```python
from build123d import *

# Parameters (mm, degrees)
F0_W          = 279.4
F0_H          = 6.35
F1_DEPTH      = 127
F1_DEPTH_BACK = 127
F2_W          = 76.2
F2_H          = 6.35
F3_DEPTH      = 82.55
F4_W          = 57.15
F4_H          = 6.35
F5_DEPTH      = 69.85
F6_R          = 1.5875
F7_DEPTH      = 6.351
F8_R          = 1.5875
F9_DEPTH      = 6.351


with BuildPart() as f1:
    # F0 (on Top) → F1 (new body, two sides)
    with BuildSketch(Plane.XY) as f1_sk:
        Rectangle(F0_W, F0_H)
    extrude(amount=F1_DEPTH)
    extrude(f1_sk.sketch, amount=-F1_DEPTH_BACK)

    # F0 (on Top) + F2 (on face) → F3 (join)
    with BuildSketch(Plane.XY):
        Rectangle(F0_W, F0_H)
    with BuildSketch(Plane.XY.offset(127)):
        Rectangle(F2_W, F2_H)
    extrude(amount=F3_DEPTH)

    # F4 (on face) → F5 (join)
    with BuildSketch(Plane(origin=(0, 0, -127), x_dir=(1, 0, 0), z_dir=(0, 0, -1))):
        Rectangle(F4_W, F4_H)
    extrude(amount=F5_DEPTH)

    # F6 (on face) → F7 (cut, through all)
    with BuildSketch(Plane.XZ.offset(3.175)):
        with Locations((-17.4625, -171.45)):
            Circle(F6_R)
        with Locations((17.4625, -171.45)):
            Circle(F6_R)
    extrude(amount=-F7_DEPTH, mode=Mode.SUBTRACT)

    # F8 (on face) → F9 (cut, through all)
    with BuildSketch(Plane.XZ.offset(3.175)):
        with Locations((-15.08125, 177.8)):
            Circle(F8_R)
        with Locations((15.08125, 177.8)):
            Circle(F8_R)
    extrude(amount=-F9_DEPTH, mode=Mode.SUBTRACT)


solid = f1.part
```
Work out the finished part from the listing and answer in its coordinate system (mm). Coordinates: 2 decimals unless noted, no trailing zeros. Order: outer loops, then holes, each group sorted by start corner. A loop starts at its lowest first (then second) coordinate and runs counter-clockwise, first axis right, second up. Notation, with made-up numbers: (28, 38) - (72, 38) arc R23 ccw to (72, 55) - close; hole circle Ø7 at (-6.5, 69.25). An arc over 180 degrees is marked (long way). Answer as a JSON object with one key per item and string values.
1. Find section B-B on x = 117.5. Determine the outline of the cut face in (y, z) (3 decimals).
Output values:
{"outline": "(-3.175, -127) - (3.175, -127) - (3.175, 127) - (-3.175, 127) - close"}
2. Find section A-A on y = -1. Count the separate pieces of the cut face and the enclosed holes in it, plus the area to 3 significant figures.
Output values:
{"separate pieces": "1", "enclosed holes": "4", "area": "81,200 mm²"}
3. Each of these flat-tipped pins is pushed along its axis until it touches: P1, Ø3, axis at x = -104, y = -1, coming from the -Z side; P2, Ø1, axis at y = 2, z = 164.5, coming from the -X side; P3, Ø1.9, axis at x = 112.5, y = 0.5, coming from the +Z side; P4, Ø3, axis at x = 15.08, z = 177.8, coming from the +Y side. Where does it stop, or does it pass through?
Output values:
{"P1": "stops at z = -127", "P2": "stops at x = -38.1", "P3": "stops at z = 127", "P4": "passes through"}
4. Consider line 1 (X direction, y = 1.25, z = -171.45) (3 decimals); line 2 (Z direction, x = 62.5, y = -0.25); line 3 (X direction, y = 0.5, z = -168.5) (3 decimals). Determine where each line is inside the solid, lowest interval first.
Output values:
{"line 1": "x = -28.575 to -19.05, -15.875 to 15.875, 19.05 to 28.575", "line 2": "z = -127 to 127", "line 3": "x = -28.575 to 28.575"}
